Geometry: final body of the model. Coordinates: model frame, mm. A direction names the side the tool comes from. Round coordinates to 2 decimals unless told otherwise and drop trailing zeros. Write each loop counter-clockwise with the first axis right and the second up, starting at its lowest first coordinate (ties: lowest second). Pieces come first, ordered by that corner, then holes. Notation, with made-up numbers: (19.5, -26.5) - (54.5, -26.5) arc R32 cw to (54.5, 0.5) - close; hole circle Ø2 at (21.5, 47). An arc over 180 degrees is marked (long way). Use a Markdown table: item, result. Add a question column.
```python
from build123d import *

# Parameters (mm, degrees)
ESQUISSE1_W             = 46.15
ESQUISSE1_H             = 34.15
BOSS_EXTRU_1_DEPTH      = 5
BOSS_EXTRU_2_DEPTH      = 3
ENL_V_MAT_EXTRU_4_DEPTH = 9
ESQUISSE7_W             = 43.35
ESQUISSE7_H             = 31.7
ENL_V_MAT_EXTRU_5_DEPTH = 7
ENL_V_MAT_EXTRU_6_DEPTH = 9


with BuildPart() as part:
    # Esquisse1 → Boss.-Extru.1 (new body)
    with BuildSketch(Plane.XY):
        Polygon((-40.258600608, 39.883341456), (44.541399392, 39.883341456), (44.541399392, 32.183341456), (52.241399392, 32.183341456), (52.241399392, -32.616658544), (44.541399392, -32.616658544), (44.541399392, -40.316658544), (-40.258600608, -40.316658544), (-40.258600608, -32.616658544), (-47.958600608, -32.616658544), (-47.958600608, 32.183341456), (-40.258600608, 32.183341456), align=None)
        with Locations((2.141399392, -0.216658544)):
            Rectangle(ESQUISSE1_W, ESQUISSE1_H, mode=Mode.SUBTRACT)
    extrude(amount=BOSS_EXTRU_1_DEPTH)

    # Esquisse2 → Boss.-Extru.2 (add)
    with BuildSketch(Plane.XY.offset(5)):
        Polygon((-47.958600608, 32.183341456), (-40.258600608, 32.183341456), (-40.258600608, 39.883341456), (44.541399392, 39.883341456), (44.541399392, 32.183341456), (52.241399392, 32.183341456), (52.241399392, -32.616658544), (44.541399392, -32.616658544), (44.541399392, -40.316658544), (-40.258600608, -40.316658544), (-40.258600608, -32.616658544), (-47.958600608, -32.616658544), align=None)
    extrude(amount=BOSS_EXTRU_2_DEPTH)

    # Esquisse6 → Enlèv. mat.-Extru.4 (cut, through all)
    with BuildSketch(Plane(origin=(0, 0, 0), x_dir=(-1, 0, 0), z_dir=(0, 0, -1))):
        with BuildLine():
            Line((-49.628899392, 29.783341456), (-44.128899392, 29.783341456))
            ThreePointArc((-44.128899392, 29.783341456), (-43.421792611, 29.490448238), (-43.128899392, 28.783341456))
            Line((-43.128899392, 28.783341456), (-43.128899392, -29.216658544))
            ThreePointArc((-43.128899392, -29.216658544), (-43.421792611, -29.923765325), (-44.128899392, -30.216658544))
            Line((-44.128899392, -30.216658544), (-49.628899392, -30.216658544))
            ThreePointArc((-49.628899392, -30.216658544), (-50.336006173, -29.923765325), (-50.628899392, -29.216658544))
            Line((-50.628899392, -29.216658544), (-50.628899392, 28.783341456))
            ThreePointArc((-50.628899392, 28.783341456), (-50.336006173, 29.490448238), (-49.628899392, 29.783341456))
        make_face()
        with BuildLine():
            Line((45.346100608, -30.216658544), (39.846100608, -30.216658544))
            ThreePointArc((39.846100608, -30.216658544), (39.138993827, -29.923765325), (38.846100608, -29.216658544))
            Line((38.846100608, -29.216658544), (38.846100608, 28.783341456))
            ThreePointArc((38.846100608, 28.783341456), (39.138993827, 29.490448238), (39.846100608, 29.783341456))
            Line((39.846100608, 29.783341456), (45.346100608, 29.783341456))
            ThreePointArc((45.346100608, 29.783341456), (46.053207389, 29.490448238), (46.346100608, 28.783341456))
            Line((46.346100608, 28.783341456), (46.346100608, -29.216658544))
            ThreePointArc((46.346100608, -29.216658544), (46.053207389, -29.923765325), (45.346100608, -30.216658544))
        make_face()
    extrude(amount=-ENL_V_MAT_EXTRU_4_DEPTH, mode=Mode.SUBTRACT)

    # Esquisse7 → Enlèv. mat.-Extru.5 (cut)
    with BuildSketch(Plane(origin=(0, 0, 5), x_dir=(-1, 0, 0), z_dir=(0, 0, -1))):
        with Locations((-2.236399392, -0.691658544)):
            Rectangle(ESQUISSE7_W, ESQUISSE7_H)
    extrude(amount=-ENL_V_MAT_EXTRU_5_DEPTH, mode=Mode.SUBTRACT)

    # Esquisse8 → Enlèv. mat.-Extru.6 (cut, through all)
    with BuildSketch(Plane(origin=(0, 0, 0), x_dir=(-1, 0, 0), z_dir=(0, 0, -1))):
        with BuildLine():
            Line((-32.141399392, 37.127856995), (27.858600608, 37.127856995))
            ThreePointArc((27.858600608, 37.127856995), (31.394134514, 35.663390901), (32.858600608, 32.127856995))
            Line((32.858600608, 32.127856995), (32.858600608, 24.127856995))
            ThreePointArc((32.858600608, 24.127856995), (31.394134514, 20.592323089), (27.858600608, 19.127856995))
            Line((27.858600608, 19.127856995), (-32.141399392, 19.127856995))
            ThreePointArc((-32.141399392, 19.127856995), (-35.676933298, 20.592323089), (-37.141399392, 24.127856995))
            Line((-37.141399392, 24.127856995), (-37.141399392, 32.127856995))
            ThreePointArc((-37.141399392, 32.127856995), (-35.676933298, 35.663390901), (-32.141399392, 37.127856995))
        make_face()
        with BuildLine():
            Line((-32.141399392, -20.511174082), (27.858600608, -20.511174082))
            ThreePointArc((27.858600608, -20.511174082), (31.394134514, -21.975640176), (32.858600608, -25.511174082))
            Line((32.858600608, -25.511174082), (32.858600608, -33.511174082))
            ThreePointArc((32.858600608, -33.511174082), (31.394134514, -37.046707988), (27.858600608, -38.511174082))
            Line((27.858600608, -38.511174082), (-32.141399392, -38.511174082))
            ThreePointArc((-32.141399392, -38.511174082), (-35.676933298, -37.046707988), (-37.141399392, -33.511174082))
            Line((-37.141399392, -33.511174082), (-37.141399392, -25.511174082))
            ThreePointArc((-37.141399392, -25.511174082), (-35.676933298, -21.975640176), (-32.141399392, -20.511174082))
        make_face()
        with BuildLine():
            Line((-43.128899392, 16.858341456), (-33.628899392, 16.858341456))
            ThreePointArc((-33.628899392, 16.858341456), (-30.093365486, 15.393875362), (-28.628899392, 11.858341456))
            Line((-28.628899392, 11.858341456), (-28.628899392, -12.141658544))
            ThreePointArc((-28.628899392, -12.141658544), (-30.093365486, -15.677192449), (-33.628899392, -17.141658544))
            Line((-33.628899392, -17.141658544), (-45.647019221, -17.141658544))
            Line((-45.647019221, -17.141658544), (-45.647019221, 16.858341456))
            Line((-45.647019221, 16.858341456), (-43.128899392, 16.858341456))
        make_face()
        with BuildLine():
            Line((41.174220437, -17.141658544), (41.174220437, 16.858341456))
            Line((41.174220437, 16.858341456), (38.656100608, 16.858341456))
            Line((38.656100608, 16.858341456), (29.156100608, 16.858341456))
            ThreePointArc((29.156100608, 16.858341456), (25.620566702, 15.393875362), (24.156100608, 11.858341456))
            Line((24.156100608, 11.858341456), (24.156100608, -12.141658544))
            ThreePointArc((24.156100608, -12.141658544), (25.620566702, -15.677192449), (29.156100608, -17.141658544))
            Line((29.156100608, -17.141658544), (41.174220437, -17.141658544))
        make_face()
    extrude(amount=-ENL_V_MAT_EXTRU_6_DEPTH, mode=Mode.SUBTRACT)


solid = part.part
```
1) Section C-C, the plane z = 2. State how many separate pieces and enclosed holes the cut face has, then the cut area to 3 significant figures.
2) Section A-A, the plane y = -8. Return the cut outline in (x, z).
3) Draft query along X for faces 5 (the flat face through (3, 15.158, 6)), 6 (the flat face through (44.541, -36, 4)), 7 (the flat face through (48, 32.183, 4)). Return one class per face: released by +X, released by -X, zero draft, split by the parting line, or undercut.
4) Material intervals for L1, parallel to Y at x = -6, z = 3.75; L2, parallel to X at y = -20, z = 2.5; L3, parallel to X at y = 3, z = 5.5, sorted ascending. Write a range as from..to.
5) Section D-D, the plane y = -27. Return the cut outline in (x, z), then the cut area to 3 significant figures.
6) Pin query (flat end, axial travel): P1, Ø2.5, axis at x = -43.5, z = 5.5, coming from the -Y side; P2, Ø6, axis at x = -20, y = 24.5, coming from the +Z side; P3, Ø2.5, axis at y = -37.5, z = 4.5, coming from the -X side. Return the tip coordinate at first contact, or that it passes through.
7) Set-up query: faces 1 (the flat face through (-40.259, 36, 4)), 2 (the flat face through (48, -32.617, 4)), 3 (the flat face through (2, 16.858, 2)), 4 (the flat face through (-24.156, 0, 4)). Return all of +Z, -Z, +X, -X, +Y, -Y with unobstructed straight access to the full face (end or side cutting, diameter ignored); none if empty.
8) Section B-B, the plane x = -5. Return the cut outline in (y, z), then the cut area to 4 significant figures.
Output values:
| question | item | result |
|---|---|---|
| 1 | separate pieces | 1 |
| 1 | enclosed holes | 5 |
| 1 | area | 1,880 mm^2 |
| 2 | outline | (-47.96, 0) - (-46.35, 0) - (-46.35, 8) - (-47.96, 8) - close; (-24.16, 0) - (-20.93, 0) - (-20.93, 5) - (-19.44, 5) - (-19.44, 8) - (-24.16, 8) - close; (23.91, 5) - (25.22, 5) - (25.22, 0) - (28.63, 0) - (28.63, 8) - (23.91, 8) - close; (50.63, 0) - (52.24, 0) - (52.24, 8) - (50.63, 8) - close |
| 3 | face 5 | undercut |
| 3 | face 6 | released by +X |
| 3 | face 7 | zero draft |
| 4 | L1 | y = -40.32..-38.51, -20.51..-17.29, 16.86..19.13, 37.13..39.88 |
| 4 | L2 | x = -47.96..-46.35, -38.85..43.13, 50.63..52.24 |
| 4 | L3 | x = -47.96..-46.35, -24.16..-19.44, 23.91..28.63, 50.63..52.24 |
| 5 | outline | (-47.96, 0) - (-46.35, 0) - (-46.35, 8) - (-47.96, 8) - close; (-38.85, 0) - (-32.86, 0) - (-32.86, 8) - (-38.85, 8) - close; (37.14, 0) - (43.13, 0) - (43.13, 8) - (37.14, 8) - close; (50.63, 0) - (52.24, 0) - (52.24, 8) - (50.63, 8) - close |
| 5 | area | 122 mm^2 |
| 6 | P1 | stops at y = -32.62 |
| 6 | P2 | passes through |
| 6 | P3 | stops at x = -40.26 |
| 7 | face 1 | +Z, -Z, -X, +Y |
| 7 | face 2 | +Z, -Z, +X, -Y |
| 7 | face 3 | -Z |
| 7 | face 4 | +Z, -Z |
| 8 | outline | (-40.32, 0) - (-38.51, 0) - (-38.51, 8) - (-40.32, 8) - close; (-20.51, 0) - (-17.29, 0) - (-17.29, 5) - (-16.54, 5) - (-16.54, 8) - (-20.51, 8) - close; (15.16, 5) - (16.86, 5) - (16.86, 0) - (19.13, 0) - (19.13, 8) - (15.16, 8) - close; (37.13, 0) - (39.88, 0) - (39.88, 8) - (37.13, 8) - close |
| 8 | area | 87.75 mm^2 |
